```python
from build123d import *

# Parameters (mm, degrees)
SKETCH_1_W                = 245
SKETCH_1_H                = 70
EXTRUDE_1_DEPTH           = 3
SKETCH_3_R                = 2
CUT_EXTRUDE_2_DEPTH       = 128.437239455
SKETCH_5_W                = 3
SKETCH_5_H                = 20
CUT_EXTRUDE_4_DEPTH       = 128.437239455
FILLET_1_R                = 1
SKETCH_6_R                = 1.5
CUT_EXTRUDE_5_DEPTH       = 128.437239455
SKETCH_7_R                = 1.5
CUT_EXTRUDE_6_DEPTH       = 128.437239455
SKETCH_8_R                = 1.5
CUT_EXTRUDE_7_DEPTH       = 128.437239455
SKETCH_9_R                = 13
CUT_EXTRUDE_8_DEPTH       = 128.437239455
SKETCH_10_R               = 2
CUT_EXTRUDE_9_DEPTH       = 128.437239455
FILLET_2_R                = 10
SKETCH_11_R               = 2.5
CUT_EXTRUDE_10_DEPTH      = 128.437239455
CUT_EXTRUDE_11_DEPTH      = 128.437239455
CUT_EXTRUDE_11_DEPTH_BACK = 128.437239455
SKETCH_12_R               = 4
SKETCH_13_R               = 1
CUT_EXTRUDE_12_DEPTH      = 128.437239455


with BuildPart() as part:
    # 草图1 → 凸台-拉伸1 (new body)
    with BuildSketch(Plane.XY):
        Rectangle(SKETCH_1_W, SKETCH_1_H)
    extrude(amount=EXTRUDE_1_DEPTH)

    # 草图3 → 切除-拉伸2 (cut, through all)
    with BuildSketch(Plane.XY.offset(3)):
        with Locations((-85.5, 15)):
            Circle(SKETCH_3_R)
        with Locations(Location((-59.5, 15, 0), (0, 0, 180))):
            Circle(SKETCH_3_R)
        with Locations((-59.5, -15)):
            Circle(SKETCH_3_R)
        with Locations(Location((-85.5, -15, 0), (0, 0, 180))):
            Circle(SKETCH_3_R)
    extrude(amount=-CUT_EXTRUDE_2_DEPTH, mode=Mode.SUBTRACT)

    # 草图5 → 切除-拉伸4 (cut, through all)
    with BuildSketch(Plane.XY.offset(3)):
        with Locations((-121, 0)):
            Rectangle(SKETCH_5_W, SKETCH_5_H)
    extrude(amount=-CUT_EXTRUDE_4_DEPTH, mode=Mode.SUBTRACT)

    # 圆角1
    fillet_1_edges = [part.edges().sort_by_distance(p)[0] for p in [
        (-122.5, -10, 1.5),
        (-122.5, 10, 1.5),
        (-122.5, -35, 1.5),
        (-122.5, 35, 1.5),
    ]]
    fillet(fillet_1_edges, radius=FILLET_1_R)

    # 草图6 → 切除-拉伸5 (cut, through all)
    with BuildSketch(Plane.XY.offset(3)):
        with Locations((-116.5, 27)):
            Circle(SKETCH_6_R)
        with Locations((-116.5, 17)):
            Circle(SKETCH_6_R)
        with Locations(Location((-116.5, -17, 0), (0, 0, 180))):
            Circle(SKETCH_6_R)
        with Locations(Location((-116.5, -27, 0), (0, 0, 180))):
            Circle(SKETCH_6_R)
    extrude(amount=-CUT_EXTRUDE_5_DEPTH, mode=Mode.SUBTRACT)

    # 草图7 → 切除-拉伸6 (cut, through all)
    with BuildSketch(Plane.XY.offset(3)):
        with Locations((-105.5, 15)):
            Circle(SKETCH_7_R)
        with Locations(Location((-105.5, -15, 0), (0, 0, 180))):
            Circle(SKETCH_7_R)
    extrude(amount=-CUT_EXTRUDE_6_DEPTH, mode=Mode.SUBTRACT)

    # 草图8 → 切除-拉伸7 (cut, through all)
    with BuildSketch(Plane.XY.offset(3)):
        with Locations((-37.5, 27)):
            Circle(SKETCH_8_R)
        with Locations((-37.5, 17)):
            Circle(SKETCH_8_R)
        with Locations(Location((-37.5, -17, 0), (0, 0, 180))):
            Circle(SKETCH_8_R)
        with Locations(Location((-37.5, -27, 0), (0, 0, 180))):
            Circle(SKETCH_8_R)
    extrude(amount=-CUT_EXTRUDE_7_DEPTH, mode=Mode.SUBTRACT)

    # 草图9 → 切除-拉伸8 (cut, through all)
    with BuildSketch(Plane.XY.offset(3)):
        with Locations((77.5, 0)):
            Circle(SKETCH_9_R)
    extrude(amount=-CUT_EXTRUDE_8_DEPTH, mode=Mode.SUBTRACT)

    # 草图10 → 切除-拉伸9 (cut, through all)
    with BuildSketch(Plane.XY.offset(3)):
        with Locations((77.5, 17.5)):
            Circle(SKETCH_10_R)
        with Locations((60, 0)):
            Circle(SKETCH_10_R)
        with Locations(Location((95, 0, 0), (0, 0, 180))):
            Circle(SKETCH_10_R)
        with Locations(Location((77.5, -17.5, 0), (0, 0, 180))):
            Circle(SKETCH_10_R)
    extrude(amount=-CUT_EXTRUDE_9_DEPTH, mode=Mode.SUBTRACT)

    # 圆角2
    fillet_2_edges = [part.edges().sort_by_distance(p)[0] for p in [
        (122.5, -35, 1.5),
        (122.5, 35, 1.5),
    ]]
    fillet(fillet_2_edges, radius=FILLET_2_R)

    # 草图11 → 切除-拉伸10 (cut, through all)
    with BuildSketch(Plane(origin=(0, 0, 0), x_dir=(-1, 0, 0), z_dir=(0, 0, -1))):
        with Locations((-114.5, 27)):
            Circle(SKETCH_11_R)
        with Locations((-14.5, 27)):
            Circle(SKETCH_11_R)
        with Locations(Location((-14.5, -27, 0), (0, 0, 180))):
            Circle(SKETCH_11_R)
        with Locations(Location((-114.5, -27, 0), (0, 0, 180))):
            Circle(SKETCH_11_R)
    extrude(amount=-CUT_EXTRUDE_10_DEPTH, mode=Mode.SUBTRACT)

    # 草图12 → 切除-拉伸11 (cut, two sides: drawn at the far end of the back side and taken through both)
    with BuildSketch(Plane(origin=(0, 0, 0), x_dir=(-1, 0, 0), z_dir=(0, 0, -1)).offset(-CUT_EXTRUDE_11_DEPTH_BACK)):
        with Locations((-59.5, 23)):
            Circle(SKETCH_12_R)
        with Locations(Location((-59.5, -23, 0), (0, 0, 180))):
            Circle(SKETCH_12_R)
    extrude(amount=CUT_EXTRUDE_11_DEPTH + CUT_EXTRUDE_11_DEPTH_BACK, mode=Mode.SUBTRACT)

    # 草图13 → 切除-拉伸12 (cut, through all)
    with BuildSketch(Plane(origin=(0, 0, 0), x_dir=(-1, 0, 0), z_dir=(0, 0, -1))):
        with Locations((-47.5, 22.6)):
            Circle(SKETCH_13_R)
        with Locations((-29.5, 22.6)):
            Circle(SKETCH_13_R)
        with Locations(Location((-29.5, -22.6, 0), (0, 0, 180))):
            Circle(SKETCH_13_R)
        with Locations(Location((-47.5, -22.6, 0), (0, 0, 180))):
            Circle(SKETCH_13_R)
    extrude(amount=-CUT_EXTRUDE_12_DEPTH, mode=Mode.SUBTRACT)


solid = part.part
```
Build history of the part. All positions in model axes, mm. Round coordinates to 2 decimals unless told otherwise and drop trailing zeros. Write each question's results on one line, items separated by ' | '. Start each with the question number.
Item 1: Mould opens along X. For faces 1 (the face through (-2, 0, 0)), 2 (the face through (63.315, -24.201, 1.521)), 3 (the face through (-61.408, 14.399, 1.521)), 4 (the face through (119.65, 31.99, 1.52)) say: pulls with the +X half, pulls with the -X half, needs draft (parallel to the pull), parting line crosses it, or undercut.
Item 2: Saw through at A-A (z = 2.5). State how many separate pieces and enclosed holes the cut face has, and give its area (3 significant figures).
Item 3: Drop a flat-ended pin along its axis: P1, Ø6, axis at x = 114.5, y = 27, coming from the -Z side. Give the stop position or say it passes through.
Item 4: Wall check: L1, parallel to Y at x = -37.5, z = 2; L2, parallel to Y at x = 77.5, z = 0.95; L3, parallel to Y at x = -105.5, z = 0.7. Give the ranges that are in metal, low to high. Write a range as [from, to].
Results are:
1) face 1: needs draft | face 2: undercut | face 3: undercut | face 4: pulls with the +X half
2) separate pieces: 1 | enclosed holes: 29 | area: 16,200 mm²
3) P1: stops at z = 0
4) L1: y = [-35, -28.5], [-25.5, -18.5], [-15.5, 15.5], [18.5, 25.5], [28.5, 35] | L2: y = [-35, -19.5], [-15.5, -13], [13, 15.5], [19.5, 35] | L3: y = [-35, -16.5], [-13.5, 13.5], [16.5, 35]
